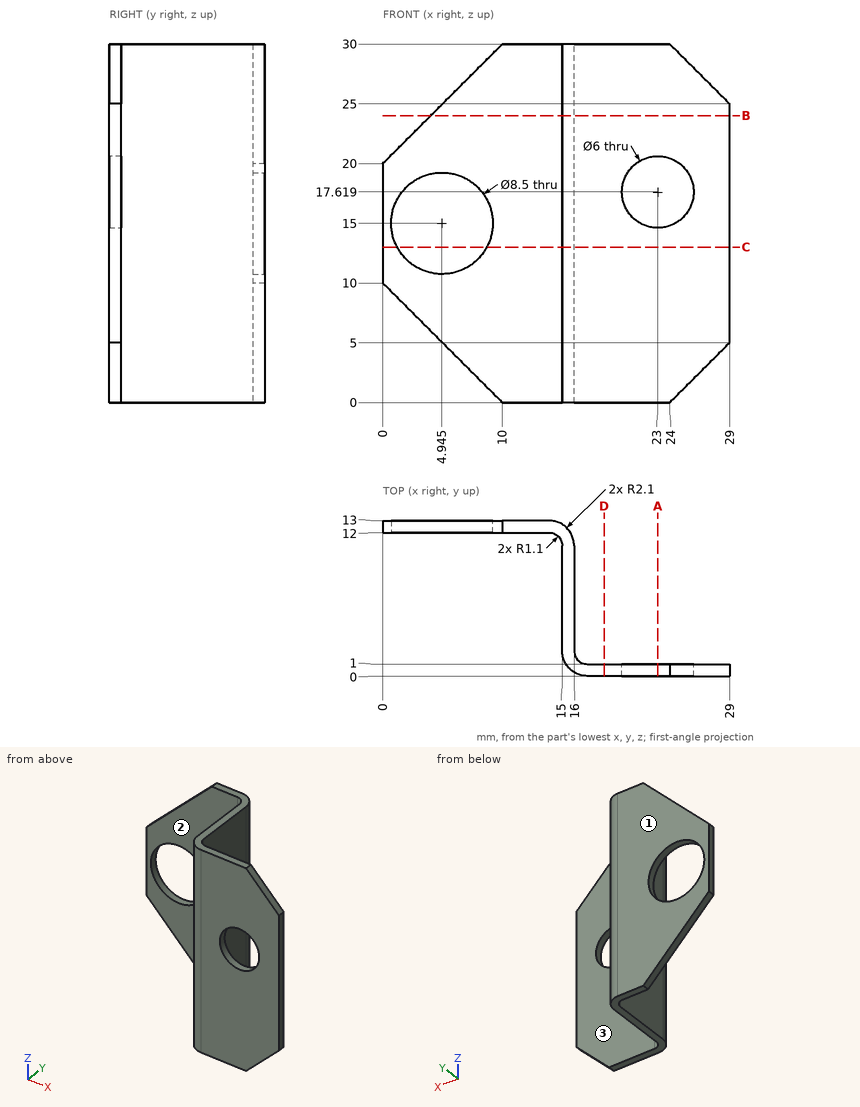
The drawing under review shows one solid part. Ordinate dimensions are in mm from its lowest x, y, z. A direction names the side the tool comes from. Round coordinates to 2 decimals unless told otherwise and drop trailing zeros. Order: outer loops, then holes, each group sorted by start corner. A loop starts at its lowest first (then second) coordinate and runs counter-clockwise, first axis right, second up. Notation, with made-up numbers: (8, 86.25) -> (53, 86.25) arc R13 cw to (53, 106.25) -> close; hole circle Ø3 at (53.25, 59.5). An arc over 180 degrees is marked (long way). Use a Markdown table: item, result.
Q1. We need section A-A on x = 23. Write out the cut boundary in (y, z), then the cut area to 3 significant figures.
Values:
| item | result |
|---|---|
| outline | (0, 0) -> (1, 0) -> (1, 14.62) -> (0, 14.62) -> close; (0, 20.62) -> (1, 20.62) -> (1, 30) -> (0, 30) -> close |
| area | 24.0 mm^2 |
Q2. Clearance check with flat-ended pins moving along their axes: P1, Ø1, axis at y = 4, z = 19, coming from the +X side; P2, Ø7, axis at x = 3.5, z = 14, coming from the -Y side; P3, Ø3.5, axis at x = 24.5, z = 17.5, coming from the +Y side. State where each tip first meets the part, or that it passes through.
Values:
| item | result |
|---|---|
| P1 | stops at x = 16 |
| P2 | stops at y = 12 |
| P3 | stops at y = 1 |
Q3. We need section B-B on z = 24. Write out the cut boundary in (x, y).
Values:
| item | result |
|---|---|
| outline | (4, 12) -> (13.9, 12) arc R1.1 cw to (15, 10.9) -> (15, 2.1) arc R2.1 ccw to (17.1, 0) -> (29, 0) -> (29, 1) -> (17.1, 1) arc R1.1 cw to (16, 2.1) -> (16, 10.9) arc R2.1 ccw to (13.9, 13) -> (4, 13) -> close |
Q4. Tool access review of the marked faces 1, 2 and 3: name each direction out of +Z, -Z, +X, -X, +Y, -Y from which nothing blocks a thin tool from reaching the whole face with its end or side.
Values:
| item | result |
|---|---|
| face 1 | +Z, -Z, +X, -X, +Y |
| face 2 | +Z, -Z, -X, -Y |
| face 3 | +Z, -Z, +X, +Y |
Q5. For line 1 (Y direction, x = 21.5, z = 3); line 2 (Y direction, x = 8.25, z = 20); line 3 (X direction, y = 5.5, z = 23), list the stretches that pass through material, from the lowest coordinate up.
Values:
| item | result |
|---|---|
| line 1 | y = 0 to 1 |
| line 2 | y = 12 to 13 |
| line 3 | x = 15 to 16 |
Q6. We need section C-C on z = 13. Write out the cut boundary in (x, y) (1 decimal).
Values:
| item | result |
|---|---|
| outline | (0, 12) -> (1.2, 12) -> (1.2, 13) -> (0, 13) -> close; (8.7, 12) -> (13.9, 12) arc R1.1 cw to (15, 10.9) -> (15, 2.1) arc R2.1 ccw to (17.1, 0) -> (29, 0) -> (29, 1) -> (17.1, 1) arc R1.1 cw to (16, 2.1) -> (16, 10.9) arc R2.1 ccw to (13.9, 13) -> (8.7, 13) -> close |
Q7. We need section D-D on x = 18.5. Write out the cut boundary in (y, z), then the cut area to 3 significant figures.
Values:
| item | result |
|---|---|
| outline | (0, 0) -> (1, 0) -> (1, 30) -> (0, 30) -> close |
| area | 30.0 mm^2 |
